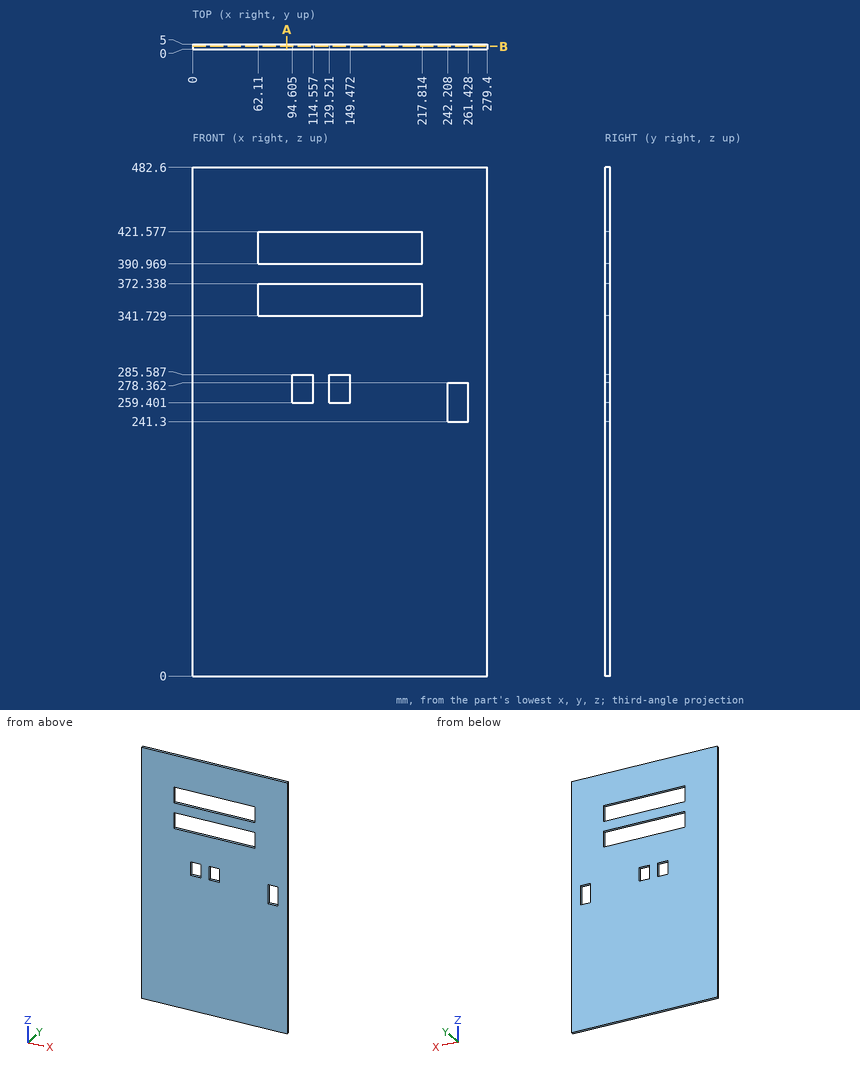
Here's the drawing with two shaded views (mm, measured from the low corner). I have some questions. Give positions to 0.01 mm unless a question says otherwise; leave off trailing zeros. Loops run counter-clockwise (first coordinate to the right, second up) from the corner with the lowest first, then second, coordinate; pieces in that order, holes last. Notation, with made-up numbers: M 46,-14.5 L 63,-14.5 A17 cw 63,-0.5 Z; hole C -24.5,17 d11. An arc over 180 degrees is marked long. Use one line per item in the form item = value. Start each with the question number.
(1) I want a section at A-A, the plane x = 89.5. Write out the boundary of the cut face in (y, z).
(2) I want a section at B-B, the plane y = 2.8. Write out the boundary of the cut face in (x, z) (1 decimal), and give its area (3 significant figures).
(3) Please list where these lines run through material, in increasing order: line 1 (Z direction, x = 135, y = 0.2); line 2 (Z direction, x = 152.5, y = 1.7); line 3 (Z direction, x = 248, y = 1.95).
Worked out:
q1.outline = M 0,0 L 5,0 L 5,341.73 L 0,341.73 Z; M 0,372.34 L 5,372.34 L 5,390.97 L 0,390.97 Z; M 0,421.58 L 5,421.58 L 5,482.6 L 0,482.6 Z
q2.outline = M 0,0 L 279.4,0 L 279.4,482.6 L 0,482.6 Z; hole M 62.1,341.7 L 217.8,341.7 L 217.8,372.3 L 62.1,372.3 Z; hole M 62.1,391 L 217.8,391 L 217.8,421.6 L 62.1,421.6 Z; hole M 94.6,259.4 L 114.6,259.4 L 114.6,285.6 L 94.6,285.6 Z; hole M 129.5,259.4 L 149.5,259.4 L 149.5,285.6 L 129.5,285.6 Z; hole M 242.2,241.3 L 261.4,241.3 L 261.4,278.4 L 242.2,278.4 Z
q2.area = 124,000 mm²
q3.line_1 = 0 to 259.4, 285.59 to 341.73, 372.34 to 390.97, 421.58 to 482.6
q3.line_2 = 0 to 341.73, 372.34 to 390.97, 421.58 to 482.6
q3.line_3 = 0 to 241.3, 278.36 to 482.6
